Source: three-view drawing plus pictorial views. Frame: mm from the lowest corner of the part. A direction names the side the tool comes from. Round coordinates to 2 decimals unless told otherwise and drop trailing zeros. Order: outer loops, then holes, each group sorted by start corner. A loop starts at its lowest first (then second) coordinate and runs counter-clockwise, first axis right, second up. Notation, with made-up numbers: (62.25, 10.5) - (83.25, 10.5) arc R4 cw to (83.25, 15.5) - close; hole circle Ø1 at (-38, 17.25). An arc over 180 degrees is marked (long way). Use one line per item in the form item = value. Start each with the question number.
Q1. Pin query (flat end, axial travel): pin 1 Ø13 at (x, y) = (20.5, 41) entering from +Z; pin 2 Ø2 at (x, y) = (32, 43.5) entering from +Z. Return the tip coordinate at first contact, or that it passes through.
Q2. Set-up query: the marked faces 1, 2 and 3. Return all of +Z, -Z, +X, -X, +Y, -Y with unobstructed straight access to the full face (end or side cutting, diameter ignored); none if empty.
Q3. Cut plane C-C, the plane y = 17. Return the cut outline in (x, z), and give its area (3 significant figures).
Q4. Cut plane D-D, the plane x = 22. Return the cut outline in (y, z), and give its area (3 significant figures).
Q5. Ray query, line 1 (Z direction, x = 22, y = 44); line 2 (Z direction, x = 29, y = 44); line 3 (Y direction, x = 29, z = 29). Return the intervals inside material, ascending. Write a range as [from, to].
Q6. Cut plane A-A, the plane x = 31.5. Return the cut outline in (y, z).
Q7. Cut plane B-B, the plane z = 13. Return the cut outline in (x, y), and give its area (3 significant figures).
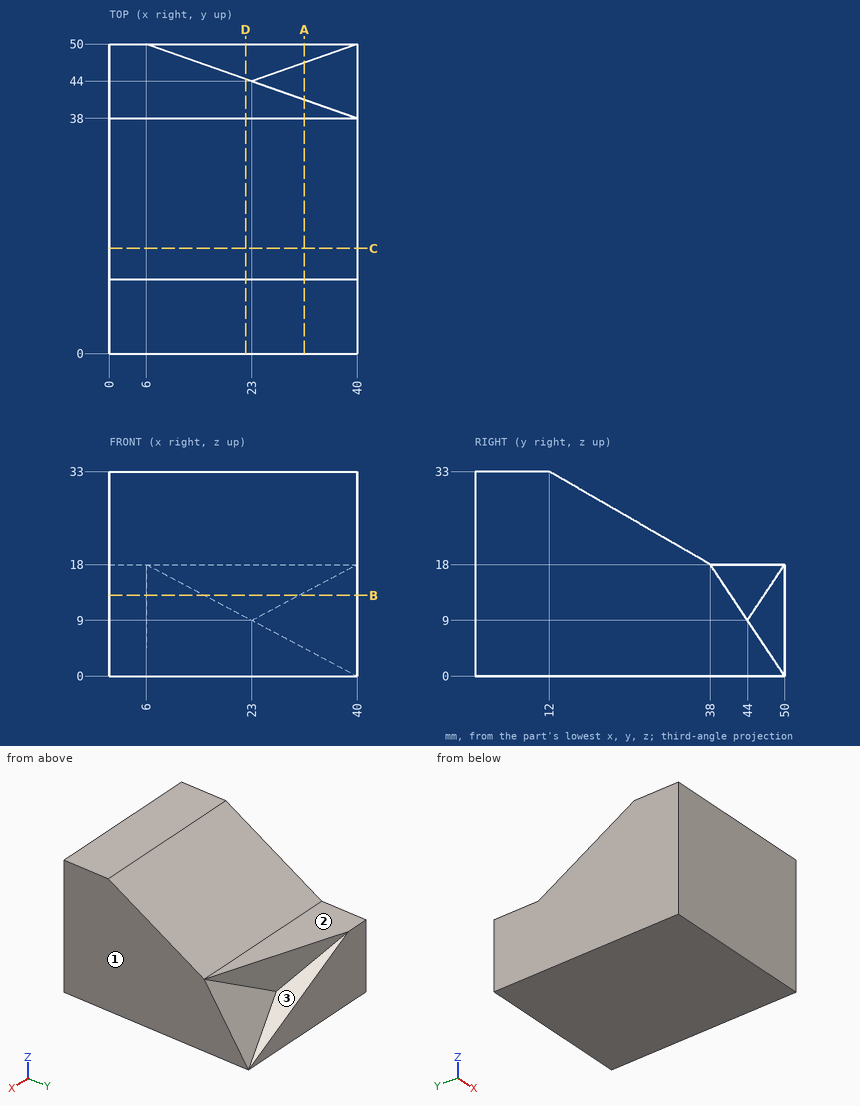
Completed:
q1.pin_1 = 20.02
q1.pin_2 = 11.25
q2.face_1 = +Z, -Z, +X, +Y, -Y
q2.face_2 = +Z, +X, -X, +Y
q2.face_3 = +Z, +X, +Y
q3.outline = (0, 0) - (40, 0) - (40, 30.12) - (0, 30.12) - close
q3.area = 1,200 mm2
q4.outline = (0, 0) - (50, 0) - (50, 9.53) - (44.35, 9.53) - (44.35, 18) - (38, 18) - (12, 33) - (0, 33) - close
q4.area = 1,230 mm2
q5.line_1 = [0, 18]
q5.line_2 = [0, 9]
q5.line_3 = [0, 18.93]
q6.outline = (0, 0) - (50, 0) - (50, 4.5) - (47, 4.5) - (41, 13.5) - (41, 18) - (38, 18) - (12, 33) - (0, 33) - close
q7.outline = (0, 0) - (40, 0) - (40, 41.33) - (30.56, 41.33) - (15.44, 46.67) - (15.44, 50) - (0, 50) - close
q7.area = 1,830 mm2
